from build123d import *

# Parameters (mm, degrees)
F0_R        = 80.899
F0_R_2      = 77.724
F1_DEPTH    = 38.1
F0_R_3      = 75.819
F0_R_4      = 73.279
F2_DEPTH    = 19.05
F3_W        = 22.7063447237
F3_H        = 49.682635814
F4_ANGLE    = 15
F5_R        = 76.3482321919
F6_DEPTH    = 16.51
F7_T2_ANGLE = 15
F9_ANGLE    = 15
F10_R       = 3.81


# Not quite as in the source:
# - a fillet or chamfer that OpenCascade refuses, or shapes differently, is made with other operations: its cross-section is extruded or revolved along the edge and cut away or added


with BuildPart() as f1:
    # F0 (on Top) → F1 (new body)
    with BuildSketch(Plane.XY):
        Circle(F0_R)
        Circle(F0_R_2, mode=Mode.SUBTRACT)
    extrude(amount=F1_DEPTH)


with BuildPart() as f1b:
    # F0 (on Top) → F1, piece 2 (new body)
    with BuildSketch(Plane.XY):
        Circle(F0_R_3)
        Circle(F0_R_4, mode=Mode.SUBTRACT)
    extrude(amount=F1_DEPTH)


with BuildPart() as f2:
    # F0 (on Top) → F2 (new body)
    with BuildSketch(Plane.XY):
        Circle(F0_R_2)
        Circle(F0_R_3, mode=Mode.SUBTRACT)
    extrude(amount=F2_DEPTH)


with BuildPart() as f4_tool:
    # F3 (on Front) → F4 (revolve)
    with BuildSketch(Plane.XZ):
        with Locations((-76.5442997217, 24.841317907)):
            Rectangle(F3_W, F3_H)
    revolve(axis=Axis((0, 0, 38.7800522149), (0, 0, -1)), revolution_arc=F4_ANGLE)


with BuildPart() as f1_1:
    add(f1.part)

    # F4: intersect by f4_tool
    add(f4_tool.part, mode=Mode.INTERSECT)



with BuildPart() as f1b_1:
    add(f1b.part)

    # F4: intersect by f4_tool
    add(f4_tool.part, mode=Mode.INTERSECT)


with BuildPart() as f2_1:
    add(f2.part)

    # F4: intersect by f4_tool
    add(f4_tool.part, mode=Mode.INTERSECT)


with BuildPart() as f6_tool:
    # F5 (on Top) → F6 (new body)
    with BuildSketch(Plane.XY):
        Circle(F5_R)
    extrude(amount=F6_DEPTH)


with BuildPart() as f1b_2:
    add(f1b_1.part)

    # F6: cut by f6_tool
    add(f6_tool.part, mode=Mode.SUBTRACT)


with BuildPart() as f2_2:
    add(f2_1.part)

    # F6: cut by f6_tool
    add(f6_tool.part, mode=Mode.SUBTRACT)

    # F7: fillet of radius 1.27 on 1 edges, made by hand

    # F7_s1 → F7_t2 (revolve)
    with BuildSketch(Plane(origin=(0, 0, 0), x_dir=(0, 0, 1), z_dir=(0.2588190451, 0.9659258263, 0))):
        with BuildLine():
            ThreePointArc((15.4784172091, -76.3482321919), (16.0581261377, -76.2082045624), (16.51, -75.819))
            Line((16.51, -75.819), (16.51, -76.3482321919))
            Line((16.51, -76.3482321919), (15.4784172091, -76.3482321919))
        make_face()
    revolve(axis=Axis((0, 0, 16.51), (0, 0, 1)), revolution_arc=F7_T2_ANGLE)


with BuildPart() as f1_2:
    add(f1_1.part)

    add(f1b_2.part)  # F9 merges F1b

    add(f2_2.part)  # F9 merges F2
    # F8 (on Front) → F9 (revolve)
    with BuildSketch(Plane.XZ):
        with BuildLine():
            ThreePointArc((-75.819, 19.939), (-76.0793820715, 19.3103820715), (-76.708, 19.05))
            Line((-76.708, 19.05), (-75.819, 19.05))
            Line((-75.819, 19.05), (-75.819, 19.939))
        make_face()
        with BuildLine():
            ThreePointArc((-76.835, 19.05), (-77.4636179285, 19.3103820715), (-77.724, 19.939))
            Line((-77.724, 19.939), (-77.724, 19.05))
            Line((-77.724, 19.05), (-76.835, 19.05))
        make_face()
    revolve(axis=Axis((0, 0, 38.7800522149), (0, 0, -1)), revolution_arc=F9_ANGLE)

    # F10
    f10_edges = [f1_2.edges().sort_by_distance(p)[0] for p in [
        (-80.206898, 10.559438, 0),
    ]]
    fillet(f10_edges, radius=F10_R)


solid = f1_2.part
Input: part model. Units: mm. Frame: model coordinates. A direction names the side the tool comes from. Coordinates: 2 decimals unless noted, no trailing zeros. Loops run counter-clockwise (first coordinate to the right, second up) from the corner with the lowest first, then second, coordinate; pieces in that order, holes last. Notation, with made-up numbers: (72.5, 23.5) -> (88.5, 23.5) arc R11 ccw to (88.5, 39.5) -> close; hole circle Ø2 at (85.5, 3). An arc over 180 degrees is marked (long way). One line per item, written item: value.
(1) Draft query along Y for faces 3 (the face through (-75.152, 10.034, 28.892)), 4 (the face through (-75.677, 10.104, 7.631)), 5 (the face through (-79, 11, 38.1)). Return one class per face: pulls with the +Y half, pulls with the -Y half, needs draft (parallel to the pull), parting line crosses it, or undercut.
Answer below:
face 3: undercut
face 4: pulls with the -Y half
face 5: needs draft
(2) Cut plane B-B (x = -72.25). Output: boundary loops of the cut face in (y, z).
Answer below:
outline: (12.24, 16.51) -> (19.36, 16.51) -> (19.36, 38.1) -> (12.24, 38.1) -> close
(3) Ray query, line 1 along Z through (x, y) = (-73.5, 16); line 2 along X through (y, z) = (16.25, 23.5); line 3 along X through (y, z) = (16, 30). Return the intervals inside material, ascending.
Answer below:
line 1: z = 16.51 to 38.1
line 2: x = -79.25 to -76.01, -74.06 to -71.45
line 3: x = -79.3 to -76.06, -74.11 to -71.51
(4) Pin query (flat end, axial travel): pin 1 Ø5 at (x, z) = (-77, 34) entering from +Y; pin 2 Ø2.5 at (x, y) = (-72.5, 12) entering from -Z; pin 3 Ø1 at (y, z) = (12.5, 21.5) entering from +X. Return the tip coordinate at first contact, or that it passes through.
Answer below:
pin 1: stops at y = 20.94
pin 2: stops at z = 16.51
pin 3: stops at x = -72.12
(5) Set-up query: faces 1 (the face through (-76, 10, 0)), 2 (the face through (-74, 10, 16.51)). Return all of +Z, -Z, +X, -X, +Y, -Y with unobstructed straight access to the full face (end or side cutting, diameter ignored); none if empty.
Answer below:
face 1: -Z, +X, -X, +Y, -Y
face 2: -Z, +X, -Y
(6) Cut plane A-A (z = 4.5). Output: boundary loops of the cut face in (x, y), then the cut area to 3 significant figures.
Answer below:
outline: (-80.9, 0) -> (-76.35, 0) arc R76.35 cw to (-73.75, 19.76) -> (-78.14, 20.94) arc R80.9 ccw to start
area: 93.7 mm2
